Here's how the part is built. I have some questions about the finished solid (model axes, mm). Coordinates: 2 decimals unless noted, no trailing zeros. Write each loop counter-clockwise with the first axis right and the second up, starting at its lowest first coordinate (ties: lowest second). Pieces come first, ordered by that corner, then holes. Notation, with made-up numbers: (33, 54) -> (41, 54) arc R12 ccw to (41, 74) -> close; hole circle Ø10 at (65.5, 43.5). An arc over 180 degrees is marked (long way). Put each result on its own line as item: value. Start each with the question number.
Item 1: I want a section at A-A, the plane z = 0. List the corners of the cut face in (x, y) for me.
Item 2: I want a section at B-B, the plane x = 0. List the corners of the cut face in (y, z) for me, then the cut area to 3 significant figures.
Item 3: I want a section at C-C, the plane y = 2.3. List the corners of the cut face in (x, z) for me, then the cut area to 3 significant figures.
Item 4: For pin 1 (1.5 mm diameter, centred on x = -48.5, y = 1.5, fed in from +Z); pin 2 (1 mm diameter, centred on x = 131, y = 3, fed in from +Z), each with a flat end and sliding along its axis, tell me the tip position at first contact or that it passes through.
Item 5: I need wall thicknesses on line 1 (X direction, y = 3.5, z = 0); line 2 (Z direction, x = -116, y = 2); line 3 (X direction, y = 1.1, z = -67). Which ranges of each line are inside material? Lowest first, please. Write a range as [from, to].
Item 6: I want a section at D-D, the plane x = 195. List the corners of the cut face in (y, z) for me, then the cut area to 3 significant figures.
from build123d import *

# Parameters (mm, degrees)
SKETCH1_R               = 241.3
SKETCH1_R_2             = 76.2
BOSS_EXTRUDE1_DEPTH     = 4.7625
F_1_4_CLEARANCE_HOLE1_D = 6.7564
F_10_CLEARANCE_HOLE1_D  = 5.1054


with BuildPart() as part:
    # Sketch1 → Boss-Extrude1 (new body)
    with BuildSketch(Plane(origin=(0, 0, 0), x_dir=(1, 0, 0), z_dir=(0, 1, 0))):
        Circle(SKETCH1_R)
        Circle(SKETCH1_R_2, mode=Mode.SUBTRACT)
    extrude(amount=BOSS_EXTRUDE1_DEPTH)

    # 1/4 Clearance Hole1 (through all)
    with Locations(Plane(origin=(0, 0, 0), x_dir=(-1, 0, 0), z_dir=(0, -1, 0))):
        with Locations((133.426417095, -141.723430894), (-133.426417095, -141.723430894), (-116.401079347, -156.009385519), (116.401079347, -156.009385519)):
            Hole(F_1_4_CLEARANCE_HOLE1_D / 2)

    # #10 Clearance Hole1 (through all)
    with Locations(Plane(origin=(0, 0, 0), x_dir=(-1, 0, 0), z_dir=(0, -1, 0))):
        with Locations((-129.594016958, 154.444135288), (129.594016958, 154.444135288)):
            Hole(F_10_CLEARANCE_HOLE1_D / 2)


solid = part.part
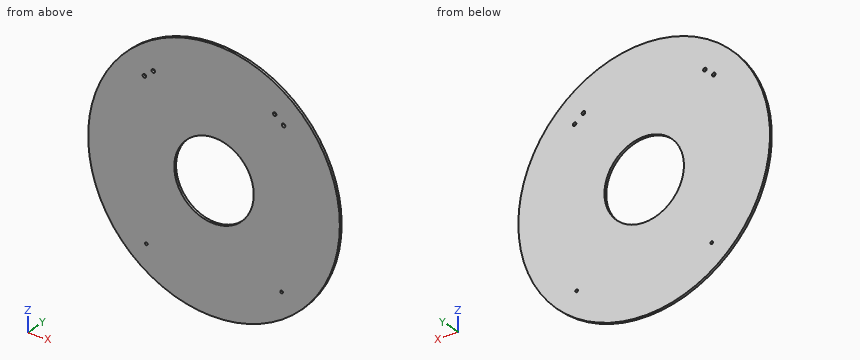
Calculated:
1. outline: (-241.3, 0) -> (-76.2, 0) -> (-76.2, 4.76) -> (-241.3, 4.76) -> close; (76.2, 0) -> (241.3, 0) -> (241.3, 4.76) -> (76.2, 4.76) -> close
2. outline: (0, -241.3) -> (4.76, -241.3) -> (4.76, -76.2) -> (0, -76.2) -> close; (0, 76.2) -> (4.76, 76.2) -> (4.76, 241.3) -> (0, 241.3) -> close
2. area: 1,570 mm2
3. outline: circle Ø482.6 at (0, 0); hole circle Ø6.76 at (-133.43, 141.72); hole circle Ø5.11 at (-129.59, -154.44); hole circle Ø6.76 at (-116.4, 156.01); hole circle Ø152.4 at (0, 0); hole circle Ø6.76 at (116.4, 156.01); hole circle Ø5.11 at (129.59, -154.44); hole circle Ø6.76 at (133.43, 141.72)
3. area: 164,000 mm2
4. pin 1: stops at z = 236.53
4. pin 2: stops at z = 202.97
5. line 1: x = [-241.3, -76.2], [76.2, 241.3]
5. line 2: z = [-211.59, 152.66], [159.36, 211.59]
5. line 3: x = [-231.81, -36.3], [36.3, 231.81]
6. outline: (0, -142.13) -> (4.76, -142.13) -> (4.76, 142.13) -> (0, 142.13) -> close
6. area: 1,350 mm2
